The listing builds one solid part. Answer for the finished solid, in the listing's coordinates (mm). A direction names the side the tool comes from. Coordinates: 2 decimals unless noted, no trailing zeros. Write each loop counter-clockwise with the first axis right and the second up, starting at its lowest first coordinate (ties: lowest second). Pieces come first, ordered by that corner, then holes.
Autodesk Inventor part; units mm, degrees
ref_plane "YZ Plane" through (0, 0, 0) normal (1, 0, 0) x (0, 1, 0)
ref_plane "XZ Plane" through (0, 0, 0) normal (0, 1, 0) x (-1, 0, 0)
ref_plane "XY Plane" through (0, 0, 0) normal (0, 0, 1) x (1, 0, 0)
sketch "Sketch1" plane through (0, 0, 0) normal (1, 0, 0) x (0, 1, 0)
  line L0 (44.4049, 39.363) -> (-19.0951, 39.363)
  line L1 (-19.0951, 39.363) -> (-19.0951, -63.507)
  line L2 (-19.0951, -63.507) -> (44.4049, -63.507)
  line L3 (44.4049, -63.507) -> (44.4049, 39.363)
  point P0 (0, 0)
  dimension "d0" = 102.87
  dimension "d1" = 63.5
extrude "Extrusion1" add sketch "Sketch1" along normal blind 5.08
sketch "Sketch2" plane through (5.08, 0, 0) normal (1, 0, 0) x (0, 0, -1)
  line L0 (63.507, 44.4049) -> (-39.363, 44.4049)
  line L1 (-39.363, 44.4049) -> (-39.363, -19.0951)
  point P0 (0, 0)
  point P1 (-34.283, 39.3249)
  point P2 (54.617, 39.3249)
  point P3 (54.617, -8.3001)
  point P4 (-34.283, -8.3001)
  dimension "d4" = 0
  dimension "d5" = 0
  dimension "d6" = 0
  dimension "d7" = 0
  dimension "d8" = 88.9
  dimension "d9" = 5.08
  dimension "d10" = 5.08
  dimension "d11" = 47.625
hole "Hole1" at (5.08, 39.3249, 34.283) at (5.08, 39.3249, -54.617) at (5.08, -8.3001, -54.617) at (5.08, -8.3001, 34.283) direction (-1, 0, 0) diameter 5.1054 end through all
fillet "Fillet1" radius 6.35 2 edges at (2.54, 44.4049, 39.363) (2.54, 44.4049, -63.507)
sketch "Sketch7" plane through (0, -19.0951, 39.363) normal (0, 0, 1) x (1, 0, 0)
  line L0 (0, 0) -> (5.08, 0)
  line L1 (5.08, 0) -> (5.08, -5.08)
  line L2 (5.08, -5.08) -> (-39.0821, -16.9132)
  line L3 (-39.0821, -16.9132) -> (-40.3969, -12.0063)
  line L4 (-40.3969, -12.0063) -> (0, -1.182)
  line L5 (0, -1.182) -> (0, 0)
  line L6 (0, 0) -> (5.08, 0)
  line L7 (0, 57.15) -> (0, 0)
  point P0 (0, 19.0951)
  dimension "d51" = 5.08
  dimension "d52" = 5.08
  dimension "d53" = 105
  dimension "d54" = 5.08
  dimension "d55" = 45.72
  dimension "d56" = 0
  dimension "d57" = 0
extrude "Extrusion4" add sketch "Sketch7" against normal blind 102.87
sketch "Sketch8" plane through (0, -20.2771, 39.363) normal (-0.258819, 0.9659258, 0) x (0.9659258, 0.258819, 0)
  line L0 (0, 0) -> (0, 102.87)
  line L1 (-41.822, 0) -> (0, 0)
  line L2 (-41.822, 102.87) -> (0, 102.87)
  point P0 (5.2481, 39.363)
  point P1 (-10.16, 25.4)
  point P2 (-35.56, 25.4)
  point P3 (-35.56, 76.2)
  point P4 (-10.16, 76.2)
  dimension "d66" = 25.4
  dimension "d67" = 0
  dimension "d68" = 25.4
  dimension "d69" = 0
  dimension "d70" = 50.8
  dimension "d71" = 0
  dimension "d72" = 0
  dimension "d73" = 26.67
hole "Hole3" at (-9.8138, -22.9067, 13.963) at (-34.3483, -29.4807, 13.963) at (-34.3483, -29.4807, -36.837) at (-9.8138, -22.9067, -36.837) direction (0.258819, -0.9659258, 0) diameter 5.1054 end through all
fillet "Fillet2" radius 6.35 2 edges at (-39.7395, -33.5549, -63.507) (-39.7395, -33.5549, 39.363)
properties part number "LimeLight120"
(1) For a pull along Y with two mould halves and no side action, classify faces 1 (the cylindrical face through (2.576, 42.495, -61.696)), 2 (the cylindrical face through (2.504, 41.817, 34.836)), 3 (the cylindrical face through (-37.9, -33.03, -61.7)) as pulls with the +Y half, pulls with the -Y half, needs draft (parallel to the pull), parting line crosses it, or undercut.
(2) Each of these flat-tipped pins is pushed along its axis until it touches: pin 1 (5 mm diameter, centred on x = -24.5, z = 26.5, fed in from -Y); pin 2 (1.5 mm diameter, centred on x = -6, z = 24.5, fed in from -Y); pin 3 (1 mm diameter, centred on x = -23, z = -48.5, fed in from +Y). Where does it stop, or does it pass through?
(3) Section D-D, the plane x = -25 is taken. Write down the section's boundary in (y, z), plus the area to 3 significant figures.
(4) Section C-C, the plane y = 13.5 is taken. Write down the section's boundary in (x, z).
(5) Which of the six approach directions +Z, -Z, +X, -X, +Y, -Y give full straight-line access (tool end or side, diameter ignored) to faces 4 (the flat face through (1, -6, 39.363)), 5 (the flat face through (0, 12, -11))?
(6) Section B-B, the plane z = -28.5 is taken. Write down the section's boundary in (x, y), plus the area to 3 significant figures.
(7) Section A-A, the plane z = 13 is taken. Write down the section's boundary in (x, y).
(8) Find the intervals of material crossed by probe 1 along X at (y, z) = (-7, -20.5); probe 2 along Y at (x, z) = (-26.5, -10); probe 3 along Y at (x, z) = (-32.5, 21), in increasing order.
Solution:
1. face 1: pulls with the +Y half
1. face 2: undercut
1. face 3: pulls with the -Y half
2. pin 1: stops at y = -32.77
2. pin 2: stops at y = -27.34
2. pin 3: stops at y = -26.31
3. outline: (-32.24, -63.51) - (-26.98, -63.51) - (-26.98, 39.36) - (-32.24, 39.36) - close
3. area: 541 mm2
4. outline: (0, -63.51) - (5.08, -63.51) - (5.08, 39.36) - (0, 39.36) - close
5. face 4: +Z, +X, -X, +Y, -Y
5. face 5: +Z, -Z, -X, +Y
6. outline: (-40.4, -31.1) - (-39.08, -36.01) - (5.08, -24.18) - (5.08, 44.4) - (0, 44.4) - (0, -20.28) - close
6. area: 561 mm2
7. outline: (-40.4, -31.1) - (-39.08, -36.01) - (-35.32, -35) - (-36.63, -30.09) - close; (-32.06, -28.87) - (-30.75, -33.78) - (-10.78, -28.43) - (-12.1, -23.52) - close; (-7.53, -22.29) - (-6.22, -27.2) - (5.08, -24.18) - (5.08, 44.4) - (0, 44.4) - (0, -20.28) - close
8. probe 1: x = 0 to 5.08
8. probe 2: y = -32.64 to -27.38
8. probe 3: y = -34.24 to -28.99
